from build123d import *

# Parameters (mm, degrees)
BOSS_EXTRUDE1_DEPTH      = 20
SKETCH2_R                = 5.1
SKETCH2_R_2              = 1.75
CUT_EXTRUDE1_DEPTH       = 79.89866919
CUT_EXTRUDE2_DEPTH       = 92.241437954
F_4_0_4_DIAMETER_HOLE1_D = 4


with BuildPart() as part:
    # Sketch1 → Boss-Extrude1 (new, symmetric)
    with BuildSketch(Plane.XY):
        Polygon((0, 0), (0, 65), (-50, 65), (-50, 55), (-10, 55), (-10, 0), align=None)
    extrude(amount=BOSS_EXTRUDE1_DEPTH, both=True)

    # Sketch2 → Cut-Extrude1 (cut, through all)
    with BuildSketch(Plane.ZY.offset(10)):
        with Locations(Location((0, 11, 0), (0, 0, 270))):
            Circle(SKETCH2_R)
        with Locations(Location((5.656854249, 16.656854249, 0), (0, 0, 270))):
            Circle(SKETCH2_R_2)
        with Locations(Location((5.656854249, 5.343145751, 0), (0, 0, 270))):
            Circle(SKETCH2_R_2)
        with Locations(Location((-5.656854249, 16.656854249, 0), (0, 0, 270))):
            Circle(SKETCH2_R_2)
        with Locations(Location((-5.656854249, 5.343145751, 0), (0, 0, 270))):
            Circle(SKETCH2_R_2)
    extrude(amount=-CUT_EXTRUDE1_DEPTH, mode=Mode.SUBTRACT)

    # Sketch3 → Cut-Extrude2 (cut, through all)
    with BuildSketch(Plane.XY.offset(20)):
        Polygon((-50, 65), (0, 65), (0, 40), (-5, 40), (-5, 30), (-10, 30), (-10, 55), (-50, 55), align=None)
    extrude(amount=-CUT_EXTRUDE2_DEPTH, mode=Mode.SUBTRACT)

    # Ø4.0 (4) Diameter Hole1 (through all)
    with Locations(Plane(origin=(0, 0, 0), x_dir=(0, 0, -1), z_dir=(1, 0, 0))):
        with Locations((-12.5, 35), (0, 35), (12.5, 35)):
            Hole(F_4_0_4_DIAMETER_HOLE1_D / 2)


solid = part.part
The model under review builds one solid part; all positions refer to its coordinate system, in mm. A direction names the side the tool comes from. Coordinates: 2 decimals unless noted, no trailing zeros. Write each loop counter-clockwise with the first axis right and the second up, starting at its lowest first coordinate (ties: lowest second). Pieces come first, ordered by that corner, then holes. Notation, with made-up numbers: (39, 59.25) - (95, 59.25) arc R12 cw to (95, 75.25) - close; hole circle Ø2 at (-2.5, 55.25). An arc over 180 degrees is marked (long way). Answer as a JSON object with one key per item and string values. Group by question number.
1. Clearance check with flat-ended pins moving along their axes: pin 1 Ø4 at (x, z) = (-8.5, 3) entering from +Y; pin 2 Ø3 at (y, z) = (16.66, 5.66) entering from -X (3 decimals); pin 3 Ø5 at (y, z) = (35, 12.5) entering from -X. State where each tip first meets the part, or that it passes through.
2. Mouldability with a two-part tool opening along Z and no side actions: class faces 3 (the face through (0, 20, 0)), 4 (the face through (-5, 20, 20)), 5 (the face through (-5.07, 6.136, 1.532)) as pulls with the +Z half, pulls with the -Z half, needs draft (parallel to the pull), parting line crosses it, or undercut.
3. Add section C-C (z = 0). Give the boundary of the cut face in (x, y), plus the area to 3 significant figures.
4. Machinability: for faces 1 (the face through (-5, 32.8, 0.3)), 2 (the face through (-5, 0, 0)), which of the approach directions +Z, -Z, +X, -X, +Y, -Y give a long, thin tool a straight path to every point of the face, cutting with its end or side? Answer none if there is none.
5. To check wall thickness, follow probe 1 along Z at (x, y) = (-4.25, 33.5); probe 2 along Z at (x, y) = (-5.75, 11); probe 3 along Z at (x, y) = (-5, 17). State the ranges of each line that lie inside material, in increasing order.
6. Add section B-B (z = -12.5). Give the boundary of the cut face in (x, y), plus the area to 3 significant figures.
7. Add section D-D (y = 4.5). Give the boundary of the cut face in (x, z).
8. Add section A-A (y = 35). Give the boundary of the cut face in (x, z), plus the area to 3 significant figures.
Findings:
{
 "1": {"pin 1": "y = 30", "pin 2": "through", "pin 3": "x = -5"},
 "2": {"face 3": "needs draft", "face 4": "pulls with the +Z half", "face 5": "undercut"},
 "3": {"outline": "(-10, 0) - (0, 0) - (0, 5.9) - (-10, 5.9) - close; (-10, 16.1) - (0, 16.1) - (0, 33) - (-5, 33) - (-5, 30) - (-10, 30) - close; (-5, 37) - (0, 37) - (0, 40) - (-5, 40) - close", "area": "228 mm²"},
 "4": {"face 1": "+Z, -Z, -X, +Y", "face 2": "+Z, -Z, +X, -X, -Y"},
 "5": {"probe 1": "-20 to -13.82, -11.18 to -1.32, 1.32 to 11.18, 13.82 to 20", "probe 2": "-20 to -5.1, 5.1 to 20", "probe 3": "-20 to -7.37, -3.94 to 3.94, 7.37 to 20"},
 "6": {"outline": "(-10, 0) - (0, 0) - (0, 33) - (-5, 33) - (-5, 30) - (-10, 30) - close; (-5, 37) - (0, 37) - (0, 40) - (-5, 40) - close", "area": "330 mm²"},
 "7": {"outline": "(-10, -20) - (0, -20) - (0, -7.19) - (-10, -7.19) - close; (-10, -4.12) - (0, -4.12) - (0, 4.12) - (-10, 4.12) - close; (-10, 7.19) - (0, 7.19) - (0, 20) - (-10, 20) - close"},
 "8": {"outline": "(-5, -20) - (0, -20) - (0, -14.5) - (-5, -14.5) - close; (-5, -10.5) - (0, -10.5) - (0, -2) - (-5, -2) - close; (-5, 2) - (0, 2) - (0, 10.5) - (-5, 10.5) - close; (-5, 14.5) - (0, 14.5) - (0, 20) - (-5, 20) - close", "area": "140 mm²"}
}
